from build123d import *

# Parameters (mm, degrees)
BOSS_EXTRUDE1_DEPTH      = 10
BOSS_EXTRUDE1_DEPTH_BACK = 10
SKETCH3_R                = 1
SKETCH3_W                = 23
SKETCH3_H                = 13
CUT_EXTRUDE1_DEPTH       = 6
SKETCH5_R                = 1
CUT_EXTRUDE2_DEPTH       = 6


with BuildPart() as part:
    # Sketch1 → Boss-Extrude1 (new body, two sides)
    with BuildSketch(Plane(origin=(0, 0, 0), x_dir=(1, 0, 0), z_dir=(0, 1, 0))) as boss_extrude1_sk:
        Polygon((0, 34.323215889), (0, 24.637864585), (15.3072, 17.5), (15.3072, -17.5), (0, -24.637864585), (0, -34.323215889), (5, -34.323215889), (5, -27.823215889), (20.3072, -20.685351304), (20.3072, 20.685351304), (5, 27.823215889), (5, 34.323215889), align=None)
    extrude(amount=BOSS_EXTRUDE1_DEPTH)
    extrude(boss_extrude1_sk.sketch, amount=-BOSS_EXTRUDE1_DEPTH_BACK)

    # Sketch3 → Cut-Extrude1 (cut, through all)
    with BuildSketch(Plane.ZY.offset(-15.3072)):
        with Locations((-13.875, 0)):
            Circle(SKETCH3_R)
        with Locations((13.875, 0)):
            Circle(SKETCH3_R)
        Rectangle(SKETCH3_W, SKETCH3_H)
    extrude(amount=-CUT_EXTRUDE1_DEPTH, mode=Mode.SUBTRACT)

    # Sketch5 → Cut-Extrude2 (cut, through all)
    with BuildSketch(Plane(origin=(5, 0, 0), x_dir=(0, 0, -1), z_dir=(1, 0, 0))):
        with Locations((31, -5)):
            Circle(SKETCH5_R)
        with Locations((31, 5)):
            Circle(SKETCH5_R)
        with Locations((-31, 5)):
            Circle(SKETCH5_R)
        with Locations((-31, -5)):
            Circle(SKETCH5_R)
    extrude(amount=-CUT_EXTRUDE2_DEPTH, mode=Mode.SUBTRACT)


solid = part.part
For this review, take the finished solid that the model builds, in its own axes (mm). A direction names the side the tool comes from. Coordinates: 2 decimals unless noted, no trailing zeros. Order: outer loops, then holes, each group sorted by start corner. A loop starts at its lowest first (then second) coordinate and runs counter-clockwise, first axis right, second up. Notation, with made-up numbers: (-26, -12) - (-7, -12) arc R18 ccw to (-7, 2) - close; hole circle Ø5 at (-22, 48.25). An arc over 180 degrees is marked (long way). Use one line per item in the form item = value.
Q1. For probe 1 along Y at (x, z) = (3.1, 31); probe 2 along X at (y, z) = (6.75, 10.5); probe 3 along Z at (x, y) = (6, -1), list the stretches that pass through material, from the lowest coordinate up. Write a range as from..to.
Checked values:
probe_1 = -10..-6, -4..4, 6..10
probe_2 = 15.31..20.31
probe_3 = -27.36..-21.84, 21.84..27.36
Q2. Consider section D-D (z = 31). Give the boundary of the cut face in (x, y).
Checked values:
outline = (0, -10) - (5, -10) - (5, -6) - (0, -6) - close; (0, -4) - (5, -4) - (5, 4) - (0, 4) - close; (0, 6) - (5, 6) - (5, 10) - (0, 10) - close
Q3. For faces 1 (the flat face through (5, 0, -31)), 2 (the flat face through (16, -10, -3)), 3 (the flat face through (7.546, 0.14, -21.119)), 4 (the flat face through (18, -6.5, 0)), 5 (the flat face through (12.546, 0.14, 24.304)), list the 3-axis set-ups (+Z, -Z, +X, -X, +Y, -Y) from which the entire face can be reached by the end or side of a thin tool; tool diameter is ignored.
Checked values:
face_1 = -Z, +X, +Y, -Y
face_2 = +Z, -Z, +X, -X, -Y
face_3 = -X, +Y, -Y
face_4 = +X, -X
face_5 = +Z, +X, +Y, -Y
Q4. For P1, Ø2.5, axis at y = 0, z = -13.875, coming from the -X side; P2, Ø3, axis at y = -5, z = 31, coming from the +X side; P3, Ø5, axis at y = -2, z = 29.5, coming from the +X side, all flat-tipped, find the tip position at first contact; note any pin that passes through.
Checked values:
P1 = 15.31
P2 = 5
P3 = 6.77
Q5. Consider section A-A (z = 4). Give the boundary of the cut face in (x, y).
Checked values:
outline = (15.31, -10) - (20.31, -10) - (20.31, -6.5) - (15.31, -6.5) - close; (15.31, 6.5) - (20.31, 6.5) - (20.31, 10) - (15.31, 10) - close
Q6. Consider section B-B (y = 5). Give the boundary of the cut face in (x, z), then the cut area to 3 significant figures.
Checked values:
outline = (0, -34.32) - (5, -34.32) - (5, -32) - (0, -32) - close; (0, -30) - (5, -30) - (5, -27.82) - (20.31, -20.69) - (20.31, -11.5) - (15.31, -11.5) - (15.31, -17.5) - (0, -24.64) - close; (0, 24.64) - (15.31, 17.5) - (15.31, 11.5) - (20.31, 11.5) - (20.31, 20.69) - (5, 27.82) - (5, 30) - (0, 30) - close; (0, 32) - (5, 32) - (5, 34.32) - (0, 34.32) - close
area = 306 mm2
Q7. Draft analysis for pull direction Z (two halves, no side actions). For faces 6 (the cylindrical face through (17.77, 0.3, -12.92)), 7 (the flat face through (2, 0, 34.323)), 8 (the flat face through (3, 0, -34.323)), state which applies: +Z half, -Z half, draft (parallel to the pull), parting line (faces both ways), or undercut.
Checked values:
face_6 = undercut
face_7 = +Z half
face_8 = -Z half
Q8. Consider section C-C (x = 1). Give the boundary of the cut face in (y, z).
Checked values:
outline = (-10, -34.32) - (10, -34.32) - (10, -24.17) - (-10, -24.17) - close; (-10, 24.17) - (10, 24.17) - (10, 34.32) - (-10, 34.32) - close; hole circle Ø2 at (-5, -31); hole circle Ø2 at (-5, 31); hole circle Ø2 at (5, -31); hole circle Ø2 at (5, 31)
